```python
from build123d import *

# Parameters (mm, degrees)
SKETCH4_R           = 7.953728713
BOSS_EXTRUDE4_DEPTH = 33.25
SKETCH5_R           = 18.3
BOSS_EXTRUDE5_DEPTH = 2.5
BOSS_EXTRUDE6_START = -27
SKETCH5_3_R         = 19.8
SKETCH5_3_R_2       = 18.3
BOSS_EXTRUDE6_DEPTH = 27
SKETCH6_R           = 15
BOSS_EXTRUDE7_DEPTH = 17.5
SKETCH7_R           = 6
BOSS_EXTRUDE8_DEPTH = 5.5
SKETCH9_R           = 3
BOSS_EXTRUDE9_DEPTH = 15
SKETCH10_R          = 1.5
CUT_EXTRUDE1_DEPTH  = 4
CIRPATTERN1_COUNT   = 6


with BuildPart() as part:
    # Sketch4 → Boss-Extrude4 (new, symmetric)
    with BuildSketch(Plane.XY):
        with Locations(Location((0, 0, 0), (0, 0, 180))):
            Circle(SKETCH4_R)
    extrude(amount=BOSS_EXTRUDE4_DEPTH, both=True)

    # Sketch5 → Boss-Extrude5 (add)
    with BuildSketch(Plane.XY.offset(30.75)):
        Circle(SKETCH5_R)
    extrude(amount=BOSS_EXTRUDE5_DEPTH)

    # Sketch5_3 → Boss-Extrude6 (add)
    # profile 1 of 2: a face of its own
    with BuildSketch(Plane.XY.offset(30.75).offset(BOSS_EXTRUDE6_START)):
        Circle(SKETCH5_3_R)
        Circle(SKETCH5_3_R_2, mode=Mode.SUBTRACT)
    # profile 2 of 2: a face of its own
    with BuildSketch(Plane.XY.offset(30.75).offset(BOSS_EXTRUDE6_START)):
        Circle(SKETCH5_3_R_2)
    extrude(amount=BOSS_EXTRUDE6_DEPTH)

    # Sketch6 → Boss-Extrude7 (add)
    with BuildSketch(Plane(origin=(0, 0, -33.25), x_dir=(-1, 0, 0), z_dir=(0, 0, -1))):
        Circle(SKETCH6_R)
    extrude(amount=-BOSS_EXTRUDE7_DEPTH)

    # Sketch7 → Boss-Extrude8 (add)
    with BuildSketch(Plane.XY.offset(33.25)):
        with Locations((0, 7)):
            Circle(SKETCH7_R)
    extrude(amount=BOSS_EXTRUDE8_DEPTH)

    # Sketch9 → Boss-Extrude9 (add)
    with BuildSketch(Plane.XY.offset(38.75)):
        with Locations((0, 7)):
            Circle(SKETCH9_R)
    extrude(amount=BOSS_EXTRUDE9_DEPTH)

    # Sketch10 → Cut-Extrude1 (cut)
    with BuildSketch(Plane.XY.offset(33.25)):
        with Locations((-15.5, 0)):
            Circle(SKETCH10_R)
    cut_extrude1 = extrude(amount=-CUT_EXTRUDE1_DEPTH, mode=Mode.SUBTRACT)

    # CirPattern1: Cut-Extrude1 ×6 about axis
    cirpattern1_axis = Axis((0, 0, 0), (0, 0, 1))
    for i in range(1, CIRPATTERN1_COUNT):
        add(cut_extrude1.rotate(cirpattern1_axis, i * 360 / CIRPATTERN1_COUNT), mode=Mode.SUBTRACT)


solid = part.part
```
Part model, mm, in its own coordinate system. A direction names the side the tool comes from. Round coordinates to 2 decimals unless told otherwise and drop trailing zeros. Write each loop counter-clockwise with the first axis right and the second up, starting at its lowest first coordinate (ties: lowest second). Pieces come first, ordered by that corner, then holes. Notation, with made-up numbers: (-29.75, 51) -> (-19.75, 51) arc R18 ccw to (-19.75, 65) -> close; hole circle Ø7 at (19.5, -12). An arc over 180 degrees is marked (long way). Return JSON: item names as keys, results as strings. Group by question number.
Q1. Saw through at D-D on z = 37.5. Write the cut outline in (x, y).
Q2. Pin check, flat tips, straight feed: pin 1 (12 mm diameter, centred on x = -7, y = -12, fed in from +Z); pin 2 (5 mm diameter, centred on x = 11, z = 5.5, fed in from -Y); pin 3 (5 mm diameter, centred on x = -6, z = -1, fed in from +Y). Stop position of each tip, or through.
Q3. Saw through at A-A on x = 0. Write the cut outline in (y, z).
Q4. Mould opens along X. For faces 4 (the cylindrical face through (17, 0, 31)), 5 (the cylindrical face through (14.985, 0.66, -24.623)), 6 (the flat face through (0, 7, 53.75)) say: pulls with the +X half, pulls with the -X half, needs draft (parallel to the pull), parting line crosses it, or undercut.
Q5. Which spindle directions (+Z, -Z, +X, -X, +Y, -Y) get a long thin tool onto all of the face, cutting with end or side? Do faces 1 (the cylindrical face through (18.9, 5.9, 17.1)), 2 (the flat face through (16, 0, 29.25)), 3 (the flat face through (9, 0, 3.75)). Say none if no direction does.
Q6. Probe L1, parallel to Z at x = 6.5, y = 12.5; L2, parallel to Y at x = -7, z = 31; L3, parallel to Y at x = 7.75, z = 31.3. List the from-to ranges inside material, lowest first. Write a range as [from, to].
Q7. Saw through at C-C on y = 14. Write the cut outline in (x, z), plus the area to 3 significant figures.
Q8. Saw through at B-B on y = 0. Write the cut outline in (x, z), plus the area to 3 significant figures.
Answer:
{
 "1": {"outline": "circle Ø12 at (0, 7)"},
 "2": {"pin 1": "z = 33.25", "pin 2": "y = -17.88", "pin 3": "y = 7.14"},
 "3": {"outline": "(-19.8, 3.75) -> (-7.95, 3.75) -> (-7.95, -15.75) -> (-15, -15.75) -> (-15, -33.25) -> (15, -33.25) -> (15, -15.75) -> (7.95, -15.75) -> (7.95, 3.75) -> (19.8, 3.75) -> (19.8, 30.75) -> (18.3, 30.75) -> (18.3, 33.25) -> (13, 33.25) -> (13, 38.75) -> (10, 38.75) -> (10, 53.75) -> (4, 53.75) -> (4, 38.75) -> (1, 38.75) -> (1, 33.25) -> (-18.3, 33.25) -> (-18.3, 30.75) -> (-19.8, 30.75) -> close"},
 "4": {"face 4": "undercut", "face 5": "parting line crosses it", "face 6": "needs draft"},
 "5": {"face 1": "+Z, -Z", "face 2": "+Z", "face 3": "none"},
 "6": {"L1": "[-33.25, -15.75], [3.75, 33.25]", "L2": "[-16.91, -14.72], [-12.12, 12.12], [14.72, 16.91]", "L3": "[-16.58, -14.92], [-11.92, 11.92], [14.92, 16.58]"},
 "7": {"outline": "(-14, 3.75) -> (14, 3.75) -> (14, 30.75) -> (11.79, 30.75) -> (11.79, 33.25) -> (9.13, 33.25) -> (9.13, 29.25) -> (6.37, 29.25) -> (6.37, 33.25) -> (-6.37, 33.25) -> (-6.37, 29.25) -> (-9.13, 29.25) -> (-9.13, 33.25) -> (-11.79, 33.25) -> (-11.79, 30.75) -> (-14, 30.75) -> close; (-5.39, -33.25) -> (5.39, -33.25) -> (5.39, -15.75) -> (-5.39, -15.75) -> close", "area": "981 mm2"},
 "8": {"outline": "(-19.8, 3.75) -> (-7.95, 3.75) -> (-7.95, -15.75) -> (-15, -15.75) -> (-15, -33.25) -> (15, -33.25) -> (15, -15.75) -> (7.95, -15.75) -> (7.95, 3.75) -> (19.8, 3.75) -> (19.8, 30.75) -> (18.3, 30.75) -> (18.3, 33.25) -> (17, 33.25) -> (17, 29.25) -> (14, 29.25) -> (14, 33.25) -> (-14, 33.25) -> (-14, 29.25) -> (-17, 29.25) -> (-17, 33.25) -> (-18.3, 33.25) -> (-18.3, 30.75) -> (-19.8, 30.75) -> close", "area": "1,970 mm2"}
}
